Part model, mm, in its own coordinate system. A direction names the side the tool comes from. Round coordinates to 2 decimals unless told otherwise and drop trailing zeros. Write each loop counter-clockwise with the first axis right and the second up, starting at its lowest first coordinate (ties: lowest second). Pieces come first, ordered by that corner, then holes. Notation, with made-up numbers: M 43,8.5 L 93,8.5 A16 ccw 93,29.5 Z; hole C 8.25,-24.5 d1. An arc over 180 degrees is marked long. One line per question, with ' | ' between items. Start each with the question number.
1) Tool access for faces 1 (the face through (-2.75, 0, 25)), 2 (the face through (1.73, 7.81, 10.35)), 3 (the face through (-3, 0, 21)), 4 (the face through (0.04, 3.89, 24.25)), 5 (the face through (-1.25, -2, 5)): list every direction of +Z, -Z, +X, -X, +Y, -Y with a clear straight run to the whole face (end or side of a thin tool).
2) Saw through at D-D (y = -6.75). List the corners of the cut face in (x, z).
3) Wall check: probe 1 along X at (y, z) = (-0.5, 26.5); probe 2 along Z at (x, y) = (0, 2.25); probe 3 along Z at (x, y) = (-3.75, 1). Give the ranges that are in metal, low to high. Write a range as [from, to].
4) Drop flat-ended pins along their axis: pin 1 Ø1 at (x, z) = (-3, 14) entering from +Y; pin 2 Ø6 at (y, z) = (0, 27) entering from -X; pin 3 Ø5 at (y, z) = (3, 24.5) entering from +X; pin 4 Ø1 at (x, y) = (4, 0.5) entering from -Z. Give the stop position or say it passes through.
5) Saw through at A-A (z = 26.5). List the corners of the cut face in (x, y), plus the area to 3 significant figures.
6) Saw through at C-C (z = 8.25). List the corners of the cut face in (x, y), plus the area to 3 significant figures.
7) Saw through at B-B (y = 0). List the corners of the cut face in (x, z).
8) Mould opens along X. For faces 6 (the face through (-0.04, -3.89, 24.25)), 7 (the face through (0, -1, 10)), 8 (the face through (0, 0, 29.5)), 9 (the face through (2.75, 0, 25)) say: pulls with the +X half, pulls with the -X half, needs draft (parallel to the pull), parting line crosses it, or undercut.
```python
from build123d import *

# Parameters (mm, degrees)
SKETCH1_R           = 8
BOSS_EXTRUDE1_DEPTH = 21
SKETCH2_W           = 2.5
SKETCH2_H           = 9
CUT_EXTRUDE1_DEPTH  = 10
SKETCH3_R           = 2
CUT_EXTRUDE2_DEPTH  = 2
BOSS_EXTRUDE2_DEPTH = 8.5
SKETCH5_R           = 1.5
CUT_EXTRUDE3_DEPTH  = 4.25


with BuildPart() as part:
    # Sketch1 → Boss-Extrude1 (new body)
    with BuildSketch(Plane.XY):
        with Locations(Location((0, 0, 0), (0, 0, 180))):
            Circle(SKETCH1_R)
    extrude(amount=BOSS_EXTRUDE1_DEPTH)

    # Sketch2 → Cut-Extrude1 (cut)
    with BuildSketch(Plane(origin=(0, 0, 0), x_dir=(-1, 0, 0), z_dir=(0, 0, -1))):
        with Locations((0, -1.5)):
            Rectangle(SKETCH2_W, SKETCH2_H)
    extrude(amount=-CUT_EXTRUDE1_DEPTH, mode=Mode.SUBTRACT)

    # Sketch3 → Cut-Extrude2 (cut)
    with BuildSketch(Plane(origin=(0, 0, 0), x_dir=(-1, 0, 0), z_dir=(0, 0, -1))):
        Circle(SKETCH3_R)
    extrude(amount=-CUT_EXTRUDE2_DEPTH, mode=Mode.SUBTRACT)

    # Sketch4 → Boss-Extrude2 (add)
    with BuildSketch(Plane.XY.offset(21)):
        with BuildLine():
            Line((-2.75, 2.75), (-2.75, -2.75))
            ThreePointArc((-2.75, -2.75), (0, -3.889087297), (2.75, -2.75))
            Line((2.75, -2.75), (2.75, 2.75))
            ThreePointArc((2.75, 2.75), (0, 3.889087297), (-2.75, 2.75))
        make_face()
    extrude(amount=BOSS_EXTRUDE2_DEPTH)

    # Sketch5 → Cut-Extrude3 (cut, symmetric)
    with BuildSketch(Plane(origin=(0, 0, 0), x_dir=(1, 0, 0), z_dir=(0, 1, 0))):
        with Locations(Location((0, -26.5, 0), (0, 0, 270))):
            Circle(SKETCH5_R)
    extrude(amount=CUT_EXTRUDE3_DEPTH, both=True, mode=Mode.SUBTRACT)


solid = part.part
```
Answer key:
1) face 1: +Z, -X, +Y, -Y | face 2: +Z, -Z | face 3: +Z | face 4: +Z, +Y | face 5: -Z
2) outline: M -4.29,0 L 4.29,0 L 4.29,21 L -4.29,21 Z
3) probe 1: x = [-2.75, -1.5], [1.5, 2.75] | probe 2: z = [10, 25], [28, 29.5] | probe 3: z = [0, 21]
4) pin 1: stops at y = 7.6 | pin 2: stops at x = -2.75 | pin 3: stops at x = 2.75 | pin 4: stops at z = 0
5) outline: M -2.75,-2.75 A3.89 ccw -1.5,-3.59 L -1.5,3.59 A3.89 ccw -2.75,2.75 Z; M 1.5,-3.59 A3.89 ccw 2.75,-2.75 L 2.75,2.75 A3.89 ccw 1.5,3.59 Z | area: 16.1 mm2
6) outline: C 0,0 d16; hole M -1.25,-6 L 1.25,-6 L 1.25,3 L -1.25,3 Z | area: 179 mm2
7) outline: M -8,0 L -2,0 L -2,2 L -1.25,2 L -1.25,10 L 1.25,10 L 1.25,2 L 2,2 L 2,0 L 8,0 L 8,21 L 2.75,21 L 2.75,29.5 L -2.75,29.5 L -2.75,21 L -8,21 Z; hole C 0,26.5 d3
8) face 6: parting line crosses it | face 7: undercut | face 8: needs draft | face 9: pulls with the +X half
